```python
from build123d import *

# Parameters (mm, degrees)
SKETCH_1_W          = 44
SKETCH_1_H          = 28
SKETCH_1_R          = 1.6
EXTRUDE_1_DEPTH     = 3
CUT_EXTRUDE_1_DEPTH = 3
FILLET_1_R          = 1.5
CHAMFER_1_SIZE      = 2


with BuildPart() as part:
    # 草图1 → 凸台-拉伸1 (new body)
    with BuildSketch(Plane.XY):
        Rectangle(SKETCH_1_W, SKETCH_1_H)
        with Locations((-19, 10)):
            Circle(SKETCH_1_R, mode=Mode.SUBTRACT)
        with Locations((-19, -10)):
            Circle(SKETCH_1_R, mode=Mode.SUBTRACT)
        with Locations((19, -10)):
            Circle(SKETCH_1_R, mode=Mode.SUBTRACT)
        with Locations((19, 10)):
            Circle(SKETCH_1_R, mode=Mode.SUBTRACT)
    extrude(amount=EXTRUDE_1_DEPTH)

    # 草图2 → 切除-拉伸1 (cut)
    with BuildSketch(Plane.XY.offset(3)):
        Polygon((-17.5, 7.51545443), (-17.5, -7.51545443), (-3.220636583, 0), align=None)
        Polygon((-12.929363417, 8.5), (0, 1.695071886), (12.929363417, 8.5), align=None)
        Polygon((0, -1.695071886), (-12.929363417, -8.5), (12.929363417, -8.5), align=None)
        Polygon((17.5, 7.51545443), (3.220636583, 0), (17.5, -7.51545443), align=None)
    extrude(amount=-CUT_EXTRUDE_1_DEPTH, mode=Mode.SUBTRACT)

    # 圆角1
    fillet_1_edges = [part.edges().sort_by_distance(p)[0] for p in [
        (0, 1.695071886, 1.5),
        (-12.929363417, 8.5, 1.5),
        (12.929363417, 8.5, 1.5),
        (-12.929363417, -8.5, 1.5),
        (0, -1.695071886, 1.5),
        (12.929363417, -8.5, 1.5),
        (3.220636583, 0, 1.5),
        (17.5, 7.51545443, 1.5),
        (17.5, -7.51545443, 1.5),
        (-17.5, 7.51545443, 1.5),
        (-17.5, -7.51545443, 1.5),
    ]]
    fillet(fillet_1_edges, radius=FILLET_1_R)

    # 倒角1
    chamfer_1_edges = [part.edges().sort_by_distance(p)[0] for p in [
        (22, -14, 1.5),
        (-22, -14, 1.5),
        (-22, 14, 1.5),
        (22, 14, 1.5),
    ]]
    chamfer(chamfer_1_edges, length=CHAMFER_1_SIZE)


solid = part.part
```
Geometry: final body of the model. Coordinates: model frame, mm. A direction names the side the tool comes from. Round coordinates to 2 decimals unless told otherwise and drop trailing zeros. Write each loop counter-clockwise with the first axis right and the second up, starting at its lowest first coordinate (ties: lowest second). Pieces come first, ordered by that corner, then holes.
Item 1: Section query B-B (y = 10). Return loops of the section in (x, z).
Item 2: Mould query, pull axis X, two halves, no side actions, for faces 1 (the face through (10.46, -3.81, 1.52)), 2 (the face through (22, 0, 1)), 3 (the face through (0, 0, 0)). Classes: +X half, -X half, draft (parallel to the pull), parting line (faces both ways), or undercut.
Item 3: Pin query (flat end, axial travel): P1, Ø1.9, axis at x = -19, y = -10, coming from the -Z side. Return the tip coordinate at first contact, or that it passes through.
Item 4: Set-up query: faces 4 (the face through (-0.01, -1.89, 1.48)), 5 (the face through (-21, -13, 1)). Return all of +Z, -Z, +X, -X, +Y, -Y with unobstructed straight access to the full face (end or side cutting, diameter ignored); none if empty.
Item 5: Section query D-D (x = 14). Return loops of the section in (y, z), plus the area to 3 significant figures.
Item 6: Section query A-A (x = -19). Return loops of the section in (y, z), plus the area to 3 significant figures.
Item 7: Material intervals for L1, parallel to Y at x = 0, z = 2.85; L2, parallel to Y at x = 19, z = 0.65; L3, parallel to Y at x = 16, z = 2.3, sorted ascending.
Item 8: Section query C-C (y = -7). Return loops of the section in (x, z).
Completed:
1. outline: (-22, 0) - (-20.6, 0) - (-20.6, 3) - (-22, 3) - close; (-17.4, 0) - (17.4, 0) - (17.4, 3) - (-17.4, 3) - close; (20.6, 0) - (22, 0) - (22, 3) - (20.6, 3) - close
2. face 1: undercut
2. face 2: +X half
2. face 3: draft
3. P1: passes through
4. face 4: +Z, -Z
4. face 5: +Z, -Z, -X, -Y
5. outline: (-14, 0) - (-5.67, 0) - (-5.67, 3) - (-14, 3) - close; (5.67, 0) - (14, 0) - (14, 3) - (5.67, 3) - close
5. area: 50.0 mm2
6. outline: (-14, 0) - (-11.6, 0) - (-11.6, 3) - (-14, 3) - close; (-8.4, 0) - (8.4, 0) - (8.4, 3) - (-8.4, 3) - close; (11.6, 0) - (14, 0) - (14, 3) - (11.6, 3) - close
6. area: 64.8 mm2
7. L1: y = -14 to -8.5, -1.89 to 1.89, 8.5 to 14
7. L2: y = -14 to -11.6, -8.4 to 8.4, 11.6 to 14
7. L3: y = -14 to -6.53, 6.53 to 14
8. outline: (-22, 0) - (-8.36, 0) - (-8.36, 3) - (-22, 3) - close; (8.36, 0) - (22, 0) - (22, 3) - (8.36, 3) - close
